Geometry: see drawing. Coordinates: mm, zero at the bounding-box minimum. Give positions to 0.01 mm unless a question says otherwise; leave off trailing zeros. Write each loop counter-clockwise with the first axis right and the second up, starting at its lowest first coordinate (ties: lowest second). Pieces come first, ordered by that corner, then holes. Notation, with made-up numbers: M -13.75,53.25 L 32.25,53.25 A29 cw 32.25,81.25 Z; hole C -30.75,26 d1. An arc over 180 degrees is marked long. Use a Markdown table: item, result. Add a question column.
(1) Material intervals for L1, parallel to Y at x = 9, z = 5.5 (1 decimal); L2, parallel to Y at x = 12.75, z = 7.5 (1 decimal); L3, parallel to X at y = 8.75, z = 3.75, sorted ascending.
(2) Pin query (flat end, axial travel): pin 1 Ø2 at (x, z) = (4, 5) entering from +Y; pin 2 Ø1.5 at (y, z) = (3, 1.5) entering from +X (1 decimal). Return the tip coordinate at first contact, or that it passes through.
(3) Draft query along Y for the marked faces 1, 2, 3 and 4. Return one class per face: released by +Y, released by -Y, zero draft, split by the parting line, or undercut.
(4) Cut plane A-A (z = 1). Output: boundary loops of the cut face in (x, y) (1 decimal), plus the area to 3 significant figures.
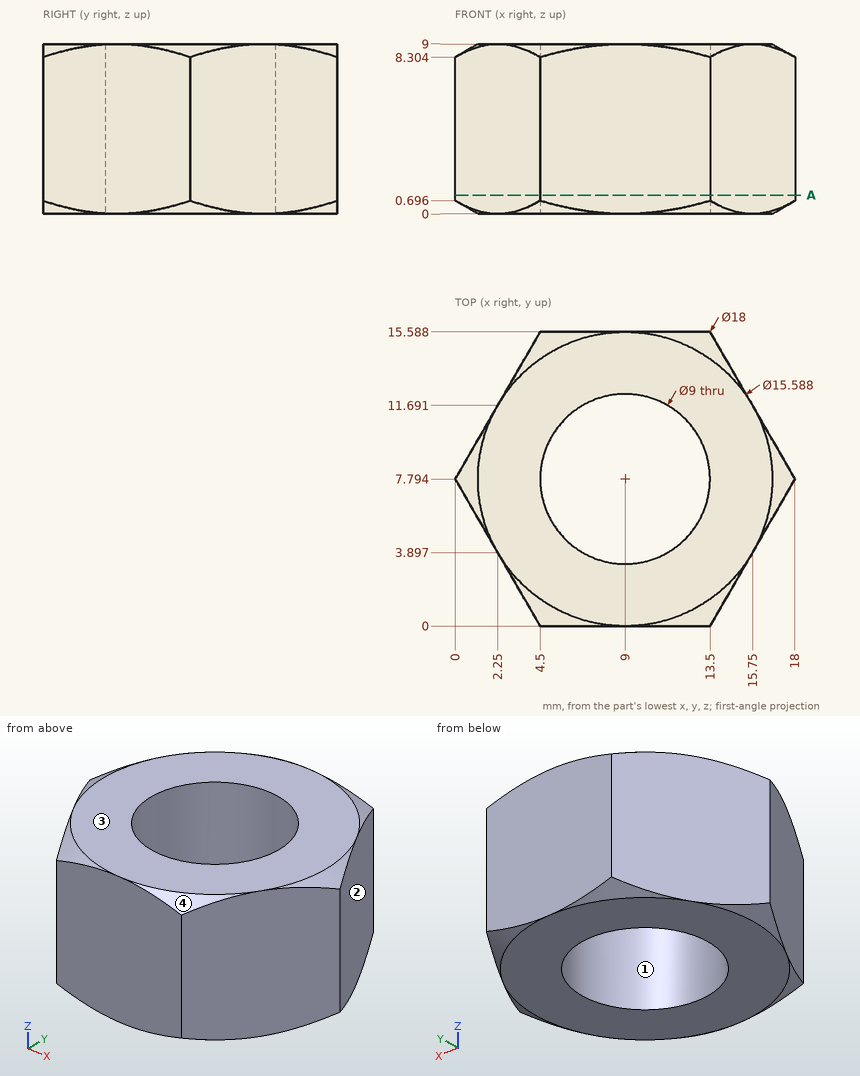
Answer list:
| question | item | result |
|---|---|---|
| 1 | L1 | 0 to 3.3, 12.3 to 15.6 |
| 1 | L2 | 0 to 5.3, 10.3 to 15.6 |
| 1 | L3 | 0.55 to 4.6, 13.4 to 17.45 |
| 2 | pin 1 | y = 15.59 |
| 2 | pin 2 | x = 15.7 |
| 3 | face 1 | undercut |
| 3 | face 2 | released by +Y |
| 3 | face 3 | zero draft |
| 3 | face 4 | released by -Y |
| 4 | outline | M 0,7.8 L 4.5,0 L 13.5,0 L 18,7.8 L 13.5,15.6 L 4.5,15.6 Z; hole C 9,7.8 d9 |
| 4 | area | 147 mm² |
